Part print with two shaded views. Sizes in mm from the minimum x, y, z corner. A direction names the side the tool comes from. Round coordinates to 2 decimals unless told otherwise and drop trailing zeros. Order: outer loops, then holes, each group sorted by start corner. A loop starts at its lowest first (then second) coordinate and runs counter-clockwise, first axis right, second up. Notation, with made-up numbers: (61.5, -11) -> (92.5, -11) arc R32 ccw to (92.5, 17) -> close; hole circle Ø1 at (6, 31). An arc over 180 degrees is marked (long way). Use a Markdown table: item, result. Add a question column.
Item 1: 3-axis set-ups, long thin cutter, end or side, ignore diameter. For the marked faces 1 and 2: which of +Z, -Z, +X, -X, +Y, -Y reach the whole face in a straight line?
Item 2: Probe L1, parallel to Y at x = 0.9, z = 12.25; L2, parallel to Z at x = 11, y = 2.5; L3, parallel to Z at x = 8.25, y = 5.25 (1 decimal). List the from-to ranges inside material, lowest first.
Item 3: Slice it at B-B, the plane x = 13.25. Give the cut face in (y, z).
Item 4: Slice it at D-D, the plane x = 18. Give the cut face in (y, z).
Item 5: Slice it at A-A, the plane z = 12.25. Give the cut face in (x, y).
Item 6: Pin check, flat tips, straight feed: pin 1 (2 mm diameter, centred on x = 7, y = 3.5, fed in from +Z); pin 2 (3 mm diameter, centred on x = 9, y = 2.5, fed in from +Z); pin 3 (3 mm diameter, centred on y = 1.5, z = 18, fed in from -X). Stop position of each tip, or through.
Item 7: Slice it at C-C, the plane y = 6.25. Give the cut face in (x, z).
Item 8: Two-plate mould, pull along Z, no slides. Class the marked faces 3, 4 and 5: released by +Z, released by -Z, zero draft, split by the parting line, or undercut.
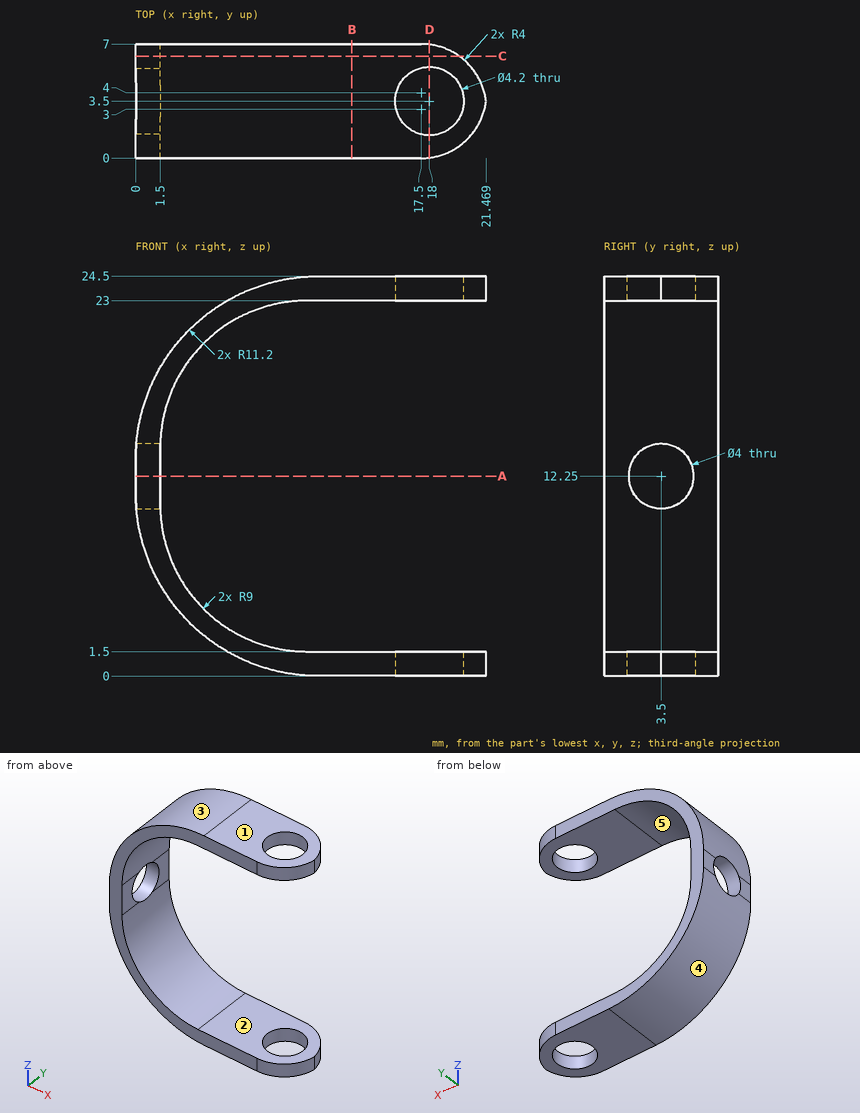
Check sheet entries:
| question | item | result |
|---|---|---|
| 1 | face 1 | +Z, +X, -X, +Y, -Y |
| 1 | face 2 | +X, +Y, -Y |
| 2 | L1 | 0 to 1.5, 5.5 to 7 |
| 2 | L2 | 0 to 1.5, 23 to 24.5 |
| 2 | L3 | 0.4 to 1.8, 22.7 to 24.1 |
| 3 | outline | (0, 0) -> (7, 0) -> (7, 1.5) -> (0, 1.5) -> close; (0, 23) -> (7, 23) -> (7, 24.5) -> (0, 24.5) -> close |
| 4 | outline | (0.03, 0) -> (1.4, 0) -> (1.4, 1.5) -> (0.03, 1.5) -> close; (0.03, 23) -> (1.4, 23) -> (1.4, 24.5) -> (0.03, 24.5) -> close; (5.6, 0) -> (6.97, 0) -> (6.97, 1.5) -> (5.6, 1.5) -> close; (5.6, 23) -> (6.97, 23) -> (6.97, 24.5) -> (5.6, 24.5) -> close |
| 5 | outline | (0, 0) -> (1.5, 0) -> (1.5, 1.5) -> (0, 1.5) -> close; (0, 5.5) -> (1.5, 5.5) -> (1.5, 7) -> (0, 7) -> close |
| 6 | pin 1 | z = 24.03 |
| 6 | pin 2 | z = 24.48 |
| 6 | pin 3 | x = 0.47 |
| 7 | outline | (0, 11.2) arc R11.2 ccw to (11.2, 0) -> (19.83, 0) -> (19.83, 1.5) -> (10.5, 1.5) arc R9 cw to (1.5, 10.5) -> (1.5, 14) arc R9 cw to (10.5, 23) -> (19.83, 23) -> (19.83, 24.5) -> (11.2, 24.5) arc R11.2 ccw to (0, 13.3) -> close |
| 8 | face 3 | released by +Z |
| 8 | face 4 | released by -Z |
| 8 | face 5 | undercut |
